Input: part model. Units: mm. Frame: model coordinates. Face numbers are marked on the shaded views. A direction names the side the tool comes from. Give positions to 0.01 mm unless a question says otherwise; leave off trailing zeros. Write each loop counter-clockwise with the first axis right and the second up, starting at its lowest first coordinate (ties: lowest second). Pieces come first, ordered by that corner, then holes.
```python
from build123d import *

# Parameters (mm, degrees)
SKETCH_1_W          = 13.5
SKETCH_1_H          = 40
EXTRUDE_1_DEPTH     = 1.5
SKETCH_1_3_W        = 1.5
SKETCH_1_3_H        = 40
EXTRUDE_2_DEPTH     = 20
SKETCH_2_W          = 13.5
SKETCH_2_H          = 1.5
EXTRUDE_3_DEPTH     = 41.5
SKETCH_3_R          = 2.75
CUT_EXTRUDE_1_DEPTH = 2
FILLET_1_R          = 1
SKETCH_10_R         = 4.4
CUT_EXTRUDE_2_DEPTH = 10
SKETCH_5_R          = 4.4
CUT_EXTRUDE_3_DEPTH = 60


with BuildPart() as part:
    # Sketch 1 → Extrude 1 (new body)
    with BuildSketch(Plane.XY):
        with Locations((6.75, -20)):
            Rectangle(SKETCH_1_W, SKETCH_1_H)
    extrude(amount=EXTRUDE_1_DEPTH)

    # Sketch 1_3 → Extrude 2 (add)
    with BuildSketch(Plane.XY):
        with Locations((14.25, -20)):
            Rectangle(SKETCH_1_3_W, SKETCH_1_3_H)
    extrude(amount=EXTRUDE_2_DEPTH)

    # Sketch 2 → Extrude 3 (add)
    with BuildSketch(Plane.XY.offset(1.5)):
        with Locations((6.75, 0.75)):
            Rectangle(SKETCH_2_W, SKETCH_2_H)
        with Locations((6.75, -40.75)):
            Rectangle(SKETCH_2_W, SKETCH_2_H)
    extrude(amount=-EXTRUDE_3_DEPTH)

    # Sketch 3 → Cut-Extrude 1 (cut)
    with BuildSketch(Plane.ZY.offset(-13.5)):
        with Locations((10, -20)):
            Circle(SKETCH_3_R)
    extrude(amount=-CUT_EXTRUDE_1_DEPTH, mode=Mode.SUBTRACT)

    # Fillet 1
    fillet_1_edges = [part.edges().sort_by_distance(p)[0] for p in [
        (14.25, 0, 20),
        (14.25, -40, 20),
        (13.5, -20, 1.5),
        (6.75, 0, 0),
        (6.75, 1.5, 1.5),
        (6.75, -40, 0),
        (15, -20, 0),
        (6.75, -41.5, 1.5),
        (13.5, 0.75, -40),
        (13.5, -40.75, -40),
        (0, -40.75, -40),
        (0, 0.75, -40),
    ]]
    fillet(fillet_1_edges, radius=FILLET_1_R)

    # Sketch 10 → Cut-Extrude 2 (cut)
    with BuildSketch(Plane.XY.offset(1.5)):
        with Locations((6.25, -20)):
            Circle(SKETCH_10_R)
    extrude(amount=-CUT_EXTRUDE_2_DEPTH, mode=Mode.SUBTRACT)

    # Sketch 5 → Cut-Extrude 3 (cut)
    with BuildSketch(Plane.XZ.offset(41.5)):
        with Locations(Location((6.75, -20, 0), (0, 0, 270))):
            Circle(SKETCH_5_R)
    extrude(amount=-CUT_EXTRUDE_3_DEPTH, mode=Mode.SUBTRACT)


solid = part.part
```
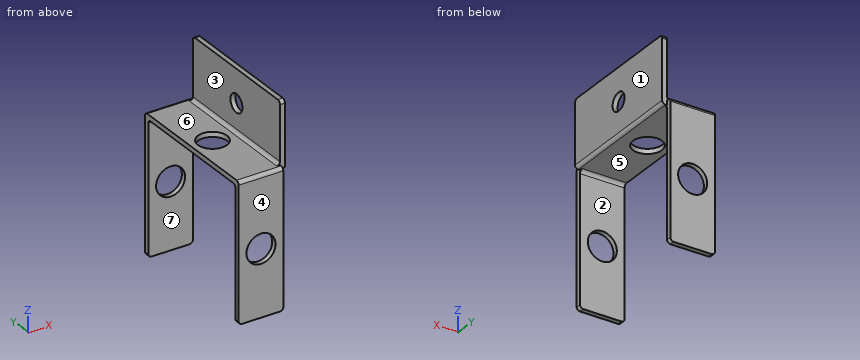
Item 1: Section B-B (y = -36). Return loops of the section in (x, z), and give its area (4 significant figures).
Item 2: Section A-A (z = 10). Return loops of the section in (x, y), and give its area (4 significant figures).
Item 3: Set-up query: the marked faces 1, 2 and 3. Return all of +Z, -Z, +X, -X, +Y, -Y with unobstructed straight access to the full face (end or side cutting, diameter ignored); none if empty.
Item 4: Section C-C (x = 9). Return loops of the section in (y, z), and give its area (3 significant figures).
Item 5: Section D-D (z = -20). Return loops of the section in (x, y), and give its area (3 significant figures).
Item 6: Ray query, line 1 (X direction, y = -40.85, z = -20); line 2 (Y direction, x = 2.5, z = -15); line 3 (X direction, y = -28, z = 17.5). Return the intervals inside material, ascending.
Item 7: Pin query (flat end, axial travel): pin 1 (2 mm diameter, centred on x = 3.5, y = -24.5, fed in from -Z); pin 2 (3 mm diameter, centred on x = 13, z = 12, fed in from -Y); pin 3 (5.5 mm diameter, centred on x = 6.25, y = -20, fed in from -Z); pin 4 (2 mm diameter, centred on x = 13, z = 5, fed in from +Y). Return the tip coordinate at first contact, or that it passes through.
Item 8: Mould query, pull axis Y, two halves, no side actions, for the marked faces 4, 5, 6 and 7. Classes: +Y half, -Y half, draft (parallel to the pull), parting line (faces both ways), or undercut.
Solved:
1. outline: (0, 0) - (14, 0) arc R1 ccw to (15, 1) - (15, 20) - (13.5, 20) - (13.5, 2.5) arc R1 cw to (12.5, 1.5) - (0, 1.5) - close
1. area: 50.25 mm2
2. outline: (13.5, -40) - (15, -40) - (15, -22.75) - (13.5, -22.75) - close; (13.5, -17.25) - (15, -17.25) - (15, 0) - (13.5, 0) - close
2. area: 51.75 mm2
3. face 1: +Z, -Z, +X, +Y, -Y
3. face 2: -Z, +X, -X
3. face 3: +Z, -X, +Y, -Y
4. outline: (-41.5, -40) - (-40, -40) - (-40, -23.78) - (-41.5, -23.78) - close; (-41.5, -16.22) - (-40, -16.22) - (-40, -1) arc R1 cw to (-39, 0) - (-23.43, 0) - (-23.43, 1.5) - (-40.5, 1.5) arc R1 ccw to (-41.5, 0.5) - close; (-16.57, 0) - (-1, 0) arc R1 cw to (0, -1) - (0, -16.22) - (1.5, -16.22) - (1.5, 0.5) arc R1 ccw to (0.5, 1.5) - (-16.57, 1.5) - close; (0, -40) - (1.5, -40) - (1.5, -23.78) - (0, -23.78) - close
4. area: 152 mm2
5. outline: (0, -41.5) - (2.35, -41.5) - (2.35, -40) - (0, -40) - close; (0, 0) - (2.35, 0) - (2.35, 1.5) - (0, 1.5) - close; (11.15, -41.5) - (13.5, -41.5) - (13.5, -40) - (11.15, -40) - close; (11.15, 0) - (13.5, 0) - (13.5, 1.5) - (11.15, 1.5) - close
5. area: 14.1 mm2
6. line 1: x = 0 to 2.35, 11.15 to 13.5
6. line 2: y = -41.5 to -40, 0 to 1.5
6. line 3: x = 13.5 to 15
7. pin 1: stops at z = 0
7. pin 2: stops at y = -40
7. pin 3: passes through
7. pin 4: stops at y = 0
8. face 4: -Y half
8. face 5: undercut
8. face 6: draft
8. face 7: undercut
